```python
from build123d import *

# Parameters (mm, degrees)
BOSS_EXTRUDE2_DEPTH = 70
SKETCH2_R           = 17.5
CUT_EXTRUDE1_DEPTH  = 70
SKETCH5_R           = 12.5
BOSS_EXTRUDE3_DEPTH = 400
FILLET3_R           = 10


with BuildPart() as part:
    # Sketch1 → Boss-Extrude2 (new body)
    with BuildSketch(Plane(origin=(0, 0, 0), x_dir=(0, 0, -1), z_dir=(1, 0, 0))):
        with BuildLine():
            Line((315, 35), (315, 47.5))
            Line((315, 47.5), (302.5, 47.5))
            Line((302.5, 47.5), (302.5, -47.5))
            Line((302.5, -47.5), (315, -47.5))
            Line((315, -47.5), (315, -35))
            Line((315, -35), (350, -35))
            ThreePointArc((350, -35), (385, 0), (350, 35))
            Line((350, 35), (315, 35))
        make_face()
    extrude(amount=BOSS_EXTRUDE2_DEPTH)

    # Sketch2 → Cut-Extrude1 (cut)
    with BuildSketch(Plane(origin=(70, 0, 0), x_dir=(0, 0, -1), z_dir=(1, 0, 0))):
        with Locations((350, 0)):
            Circle(SKETCH2_R)
    extrude(amount=-CUT_EXTRUDE1_DEPTH, mode=Mode.SUBTRACT)

    # Sketch5 → Boss-Extrude3 (add)
    with BuildSketch(Plane.XY.offset(-302.5)):
        with Locations((35, 0)):
            Circle(SKETCH5_R)
    extrude(amount=BOSS_EXTRUDE3_DEPTH)

    # Fillet3
    fillet3_edges = [part.edges().sort_by_distance(p)[0] for p in [
        (22.5, 0, 97.5),
    ]]
    fillet(fillet3_edges, radius=FILLET3_R)


solid = part.part
```
Source: CAD feature listing. Evaluate the final solid. Frame: model axes, mm. A direction names the side the tool comes from. Round coordinates to 2 decimals unless told otherwise and drop trailing zeros. Loops run counter-clockwise (first coordinate to the right, second up) from the corner with the lowest first, then second, coordinate; pieces in that order, holes last.
1. Section query B-B on z = -208.5. Output: boundary loops of the cut face in (x, y), and give its area (3 significant figures).
2. Mould query, pull axis Y, two halves, no side actions, for faces 4 (the flat face through (35, -47.5, -309)), 5 (the flat face through (70, 11, -334)), 6 (the cylindrical face through (35.49, 5.26, -366.69)). Classes: released by +Y, released by -Y, zero draft, split by the parting line, or undercut.
3. Contact query for flat-ended pins moving along their axis: pin 1 (14 mm diameter, centred on x = 18, y = 44, fed in from -Z); pin 2 (10 mm diameter, centred on y = 12.5, z = -223.5, fed in from +X); pin 3 (1.5 mm diameter, centred on x = 25, y = 28, fed in from -Z). Output: stop coordinate, or through.
4. Ray query, L1, parallel to Y at x = 41.5, z = -350; L2, parallel to Z at x = 19.5, y = -1; L3, parallel to Y at x = 45, z = -335.5. Return the intervals inside material, ascending.
5. Section query C-C on y = -21.5. Output: boundary loops of the cut face in (x, z).
6. Access query for faces 1 (the cylindrical face through (22.512, 0.55, -110.23)), 2 (the flat face through (35, 35, -333)), 3 (the flat face through (35, -35, -332)). Directions: +Z, -Z, +X, -X, +Y, -Y. A direction counts if a zero-diameter tool reaches every point of the face in a straight line with its end or side. Return the directions, or none.
7. Section query A-A on z = -338.5. Output: boundary loops of the cut face in (x, y), and give its area (3 significant figures).
Answers below:
1. outline: circle Ø25 at (35, 0)
1. area: 491 mm2
2. face 4: released by -Y
2. face 5: zero draft
2. face 6: undercut
3. pin 1: stops at z = -315
3. pin 2: stops at x = 45
3. pin 3: stops at z = -371.96
4. L1: y = -35 to -17.5, 17.5 to 35
4. L2: z = -384.99 to -367.47, -332.53 to -302.5
4. L3: y = -35 to -9.8, 9.8 to 35
5. outline: (0, -377.62) - (70, -377.62) - (70, -302.5) - (0, -302.5) - close
6. face 1: +Z
6. face 2: -Z, +X, -X, +Y
6. face 3: -Z, +X, -X, -Y
7. outline: (0, -35) - (70, -35) - (70, -13.19) - (0, -13.19) - close; (0, 13.19) - (70, 13.19) - (70, 35) - (0, 35) - close
7. area: 3,050 mm2
